The model under review builds one solid part; all positions refer to its coordinate system, in mm. Face numbers are marked on the shaded views. A direction names the side the tool comes from. Give positions to 0.01 mm unless a question says otherwise; leave off trailing zeros. Order: outer loops, then holes, each group sorted by start corner. A loop starts at its lowest first (then second) coordinate and runs counter-clockwise, first axis right, second up.
```python
from build123d import *

# Parameters (mm, degrees)
SKETCH1_R           = 9.67330264
BOSS_EXTRUDE1_DEPTH = 1
SKETCH2_R           = 8.112606278
BOSS_EXTRUDE2_DEPTH = 15
SKETCH3_R           = 9.572114115
BOSS_EXTRUDE3_DEPTH = 2
SKETCH4_R           = 8.298124112
CUT_EXTRUDE2_DEPTH  = 1
SKETCH5_R           = 2.945552355
CUT_EXTRUDE3_DEPTH  = 1


with BuildPart() as part:
    # Sketch1 → Boss-Extrude1 (new body)
    with BuildSketch(Plane(origin=(0, 0, 0), x_dir=(1, 0, 0), z_dir=(0, 1, 0))):
        with Locations(Location((0, 0, 0), (0, 0, 270))):
            Circle(SKETCH1_R)
    extrude(amount=BOSS_EXTRUDE1_DEPTH)

    # Sketch2 → Boss-Extrude2 (add)
    with BuildSketch(Plane(origin=(0, 1, 0), x_dir=(1, 0, 0), z_dir=(0, 1, 0))):
        with Locations(Location((0, 0, 0), (0, 0, 270))):
            Circle(SKETCH2_R)
    extrude(amount=BOSS_EXTRUDE2_DEPTH)

    # Sketch3 → Boss-Extrude3 (add)
    with BuildSketch(Plane(origin=(0, 16, 0), x_dir=(1, 0, 0), z_dir=(0, 1, 0))):
        with Locations(Location((0, 0, 0), (0, 0, 270))):
            Circle(SKETCH3_R)
    extrude(amount=BOSS_EXTRUDE3_DEPTH)

    # Sketch4 → Cut-Extrude2 (cut)
    with BuildSketch(Plane(origin=(0, 18, 0), x_dir=(1, 0, 0), z_dir=(0, 1, 0))):
        with Locations(Location((0, 0, 0), (0, 0, 270))):
            Circle(SKETCH4_R)
    extrude(amount=-CUT_EXTRUDE2_DEPTH, mode=Mode.SUBTRACT)

    # Sketch5 → Cut-Extrude3 (cut)
    with BuildSketch(Plane(origin=(0, 17, 0), x_dir=(1, 0, 0), z_dir=(0, 1, 0))):
        with Locations(Location((0, 0, 0), (0, 0, 270))):
            Circle(SKETCH5_R)
    extrude(amount=-CUT_EXTRUDE3_DEPTH, mode=Mode.SUBTRACT)


solid = part.part
```
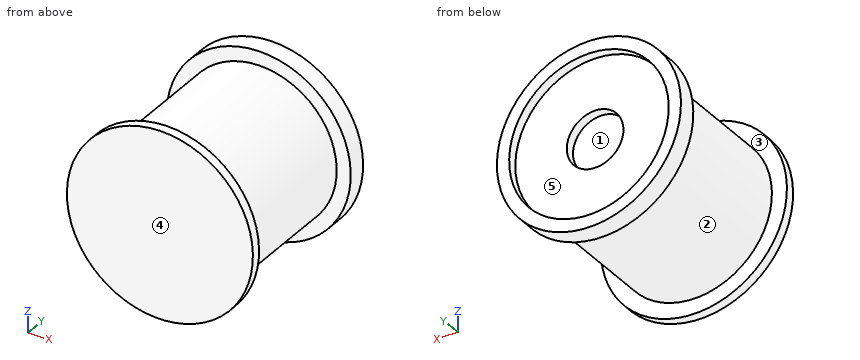
Item 1: Take a section at C-C (y = 2.75). Give the boundary of the cut face in (x, z).
Values found:
outline: circle Ø16.23 at (0, 0)
Item 2: Take a section at A-A (x = 0). Give the boundary of the cut face in (y, z).
Values found:
outline: (0, -9.67) - (1, -9.67) - (1, -8.11) - (16, -8.11) - (16, -9.57) - (18, -9.57) - (18, -8.3) - (17, -8.3) - (17, -2.95) - (16, -2.95) - (16, 2.95) - (17, 2.95) - (17, 8.3) - (18, 8.3) - (18, 9.57) - (16, 9.57) - (16, 8.11) - (1, 8.11) - (1, 9.67) - (0, 9.67) - close
Item 3: For the marked faces 1 and 2, list the 3-axis set-ups (+Z, -Z, +X, -X, +Y, -Y) from which the entire face can be reached by the end or side of a thin tool; tool diameter is ignored.
Values found:
face 1: +Y
face 2: none
Item 4: Clearance check with flat-ended pins moving along their axes: pin 1 Ø3 at (x, z) = (-0.5, 1.5) entering from +Y; pin 2 Ø4 at (x, y) = (-1, 12) entering from -Z; pin 3 Ø6 at (y, z) = (5.5, 3) entering from +X. State where each tip first meets the part, or that it passes through.
Values found:
pin 1: stops at y = 17
pin 2: stops at z = -8.11
pin 3: stops at x = 8.11
Item 5: Take a section at D-D (x = -4). Give the boundary of the cut face in (y, z).
Values found:
outline: (0, -8.81) - (1, -8.81) - (1, -7.06) - (16, -7.06) - (16, -8.7) - (18, -8.7) - (18, -7.27) - (17, -7.27) - (17, 7.27) - (18, 7.27) - (18, 8.7) - (16, 8.7) - (16, 7.06) - (1, 7.06) - (1, 8.81) - (0, 8.81) - close
Item 6: Take a section at B-B (z = 0). Give the boundary of the cut face in (x, y).
Values found:
outline: (-9.67, 0) - (9.67, 0) - (9.67, 1) - (8.11, 1) - (8.11, 16) - (9.57, 16) - (9.57, 18) - (8.3, 18) - (8.3, 17) - (2.95, 17) - (2.95, 16) - (-2.95, 16) - (-2.95, 17) - (-8.3, 17) - (-8.3, 18) - (-9.57, 18) - (-9.57, 16) - (-8.11, 16) - (-8.11, 1) - (-9.67, 1) - close
Item 7: Draft analysis for pull direction Y (two halves, no side actions). For the marked faces 3, 4 and 5, state which applies: released by +Y, released by -Y, zero draft, split by the parting line, or undercut.
Values found:
face 3: undercut
face 4: released by -Y
face 5: released by +Y
Item 8: For line 1 (Y direction, x = 1.25, z = -8.5); line 2 (X direction, y = 17.7, z = 0); line 3 (X direction, y = 16.7, z = 0), list the stretches that pass through material, from the lowest coordinate up.
Values found:
line 1: y = 0 to 1, 16 to 18
line 2: x = -9.57 to -8.3, 8.3 to 9.57
line 3: x = -9.57 to -2.95, 2.95 to 9.57
